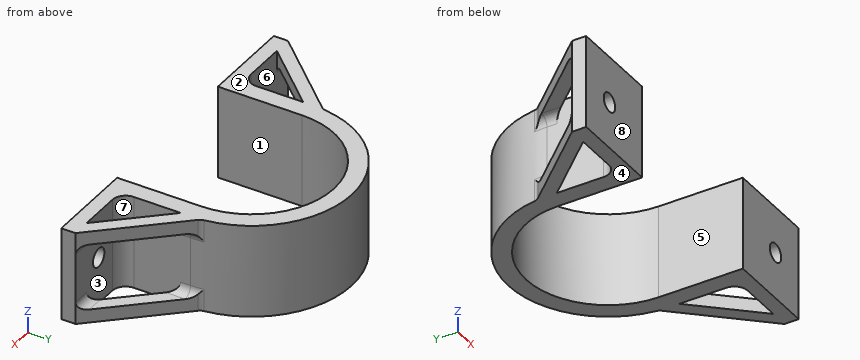
Autodesk Inventor part; units mm, degrees
ref_plane "YZ Plane" through (0, 0, 0) normal (1, 0, 0) x (0, 1, 0)
ref_plane "XZ Plane" through (0, 0, 0) normal (0, 1, 0) x (-1, 0, 0)
ref_plane "XY Plane" through (0, 0, 0) normal (0, 0, 1) x (1, 0, 0)
sketch "Эскиз1" plane through (0, 0, 0) normal (0, 0, 1) x (1, 0, 0)
  arc A0 (18.5, 0) -> (-18.5, 0) centre (0, 0) ccw
  line L0 (-22.5, 0) -> (22.5, 0)
  arc A1 (22.5, 0) -> (-22.5, 0) centre (0, 0) ccw
  line L1 (-22.5, 0) -> (-22.5, -12.8)
  line L2 (-22.5, -19) -> (-35.5, -19)
  line L3 (-35.5, -19) -> (-35.5, -15.8)
  line L4 (-35.5, -15.8) -> (-25.5, -15.8)
  arc A2 (-25.5, -15.8) -> (-22.5, -12.8) centre (-25.5, -12.8) ccw
  line L5 (-18.5, 0) -> (-18.5, -19)
  line L6 (-18.5, -19) -> (-22.5, -19)
  line L7 (0, 0) -> (0, 6.7823)
  line L8 (22.5, 0) -> (22.5, -12.8)
  line L9 (22.5, -19) -> (35.5, -19)
  line L10 (35.5, -19) -> (35.5, -15.8)
  line L11 (35.5, -15.8) -> (25.5, -15.8)
  arc A3 (22.5, -12.8) -> (25.5, -15.8) centre (25.5, -12.8) ccw
  line L12 (18.5, 0) -> (18.5, -19)
  line L13 (18.5, -19) -> (22.5, -19)
  dimension "d0" = 37
  dimension "d1" = 45
  dimension "d2" = 13
  dimension "d3" = 3.2
  dimension "d4" = 3
extrude "Выдавливание1" add sketch "Эскиз1" along normal blind 15 contours A0 L0 A1 | L0 L8 A3 L11 L10 L9 L13 L12 | L5 L6 L2 L3 L4 A2 L1 L0
sketch "Эскиз2" plane through (-35.5, -15.8, 0) normal (0, 1, 0) x (1, 0, 0)
  line L0 (71, 0) -> (61, 0)
  line L1 (61, 0) -> (61, -15)
  line L2 (71, -15) -> (61, -15)
  line L3 (71, 0) -> (71, -15)
  line L4 (71, -7.5) -> (0, -7.5)
  line L5 (0, 0) -> (0, -15)
  line L6 (10, 0) -> (0, 0)
  line L7 (10, 0) -> (10, -15)
  line L8 (10, -15) -> (0, -15)
  line L9 (5, -15) -> (5, 0)
  circle A0 centre (5, -7.5) radius 2.1
  line L10 (35.5, 0) -> (35.5, -25.4)
  circle A1 centre (66, -7.5) radius 2.1
  dimension "d7" = 4.2
extrude "Выдавливание2" cut sketch "Эскиз2" against normal blind 20 contours A1 L4 | L4 A1 | A0 L9 L4 | L4 L9 A0 | L9 A0 L4 | L4 A0 L9
sketch "Эскиз3" plane through (0, 0, 15) normal (0, 0, 1) x (1, 0, 0)
  line L0 (35.5, -15.8) -> (39.0359, -15.8)
  line L1 (22.5, 0) -> (37, -15.8)
  line L2 (21.3948, -1.0142) -> (35.8948, -16.8142)
  line L3 (22.3766, 2.3529) -> (39.0359, -15.8)
  line L4 (-18.5, -19) -> (-18.5, 0)
  arc A0 (18.5, 0) -> (-18.5, 0) centre (0, 0) ccw
  line L5 (18.5, 0) -> (18.5, -19)
  line L6 (18.5, -19) -> (35.5, -19)
  line L7 (35.5, -19) -> (35.5, -15.8)
  line L8 (35.5, -15.8) -> (25.5, -15.8)
  arc A1 (22.5, -12.8) -> (25.5, -15.8) centre (25.5, -12.8) ccw
  line L9 (22.5, -12.8) -> (22.5, 0)
  arc A2 (22.5, 0) -> (-22.5, 0) centre (0, 0) ccw
  line L10 (-22.5, 0) -> (-22.5, -12.8)
  arc A3 (-25.5, -15.8) -> (-22.5, -12.8) centre (-25.5, -12.8) ccw
  line L11 (-25.5, -15.8) -> (-35.5, -15.8)
  line L12 (-35.5, -15.8) -> (-35.5, -19)
  line L13 (-35.5, -19) -> (-18.5, -19)
  line L14 (39.0359, -15.8) -> (35.5, -15.8)
  line L15 (35.5, -15.8) -> (35.5, -19)
  line L16 (35.5, -19) -> (39.0359, -19)
  line L17 (39.0359, -19) -> (39.0359, -15.8)
  line L18 (0, 0) -> (0, 30.1625)
  line L19 (-35.5, -15.8) -> (-39.0359, -15.8)
  line L20 (-22.5, 0) -> (-37, -15.8)
  line L21 (-21.3948, -1.0142) -> (-35.8948, -16.8142)
  line L22 (-22.3766, 2.3529) -> (-39.0359, -15.8)
  line L23 (-18.5, 0) -> (-18.5, -19)
  line L24 (-18.5, -19) -> (-35.5, -19)
  line L25 (-35.5, -19) -> (-35.5, -15.8)
  line L26 (-35.5, -15.8) -> (-25.5, -15.8)
  arc A4 (-25.5, -15.8) -> (-22.5, -12.8) centre (-25.5, -12.8) ccw
  line L27 (-22.5, -12.8) -> (-22.5, 0)
  line L28 (-39.0359, -15.8) -> (-35.5, -15.8)
  line L29 (-35.5, -15.8) -> (-35.5, -19)
  line L30 (-35.5, -19) -> (-39.0359, -19)
  line L31 (-39.0359, -19) -> (-39.0359, -15.8)
  point P0 (22.5, -2.2185)
  point P1 (34.9641, -15.8)
  point P2 (35.5, -16.384)
  point P3 (-34.9641, -15.8)
  point P4 (-22.5, -2.2185)
  dimension "d11" = 1.5
  dimension "d12" = 1.5
extrude "Выдавливание3" add sketch "Эскиз3" along normal blind 3 contours L8 L2 L9 L1 L0 | L0 L17 L16 L7 | L7 L2 L8 | L1 A2 L3 L0 | L7 L6 L5 A0 L18 A2 L9 A1 L8 L2 | L18 A0 L4 L13 L12 L21 L11 A3 L10 A2 | A2 L20 L19 L22 | L10 L21 L11 L19 L20 | L19 L12 L30 L31 | L21 L12 L11
sketch "Эскиз4" plane through (0, 0, 0) normal (0, 0, -1) x (-1, 0, 0)
  line L0 (18.5, -19) -> (18.5, 0)
  line L1 (35.5, -19) -> (18.5, -19)
  line L2 (35.5, -15.8) -> (35.5, -19)
  line L3 (25.5, -15.8) -> (35.5, -15.8)
  arc A0 (22.5, -12.8) -> (25.5, -15.8) centre (25.5, -12.8) ccw
  line L4 (22.5, 0) -> (22.5, -12.8)
  arc A1 (22.5, 0) -> (-22.5, 0) centre (0, 0) ccw
  line L5 (-22.5, -12.8) -> (-22.5, 0)
  arc A2 (-25.5, -15.8) -> (-22.5, -12.8) centre (-25.5, -12.8) ccw
  line L6 (-35.5, -15.8) -> (-25.5, -15.8)
  line L7 (-35.5, -19) -> (-35.5, -15.8)
  line L8 (-18.5, -19) -> (-35.5, -19)
  line L9 (-18.5, 0) -> (-18.5, -19)
  arc A3 (18.5, 0) -> (-18.5, 0) centre (0, 0) ccw
  line L10 (-35.5, -19) -> (-35.5, -15.8)
  line L11 (-35.5, -15.8) -> (-34.9641, -15.8)
  line L12 (-22.5, -2.2185) -> (-34.9641, -15.8)
  line L13 (-22.5, -2.2185) -> (-22.5, 0)
  arc A4 (-22.3766, 2.3529) -> (-22.5, 0) centre (0, 0) ccw
  line L14 (-39.0359, -15.8) -> (-22.3766, 2.3529)
  line L15 (-39.0359, -19) -> (-39.0359, -15.8)
  line L16 (-35.5, -19) -> (-39.0359, -19)
  line L17 (35.5, -15.8) -> (35.5, -19)
  line L18 (39.0359, -19) -> (35.5, -19)
  line L19 (39.0359, -15.8) -> (39.0359, -19)
  line L20 (22.3766, 2.3529) -> (39.0359, -15.8)
  arc A5 (22.5, 0) -> (22.3766, 2.3529) centre (0, 0) ccw
  line L21 (22.5, 0) -> (22.5, -2.2185)
  line L22 (34.9641, -15.8) -> (22.5, -2.2185)
  line L23 (34.9641, -15.8) -> (35.5, -15.8)
  point P0 (-22.3766, 2.3529)
extrude "Выдавливание4" add sketch "Эскиз4" along normal blind 3 contours L0 A3 L9 L8 L7 L6 A2 L5 A1 L4 A0 L3 L2 L1 | L2 L3 L22 L4 A1 L20 L19 L18 | L16 L15 L14 A1 L5 L12 L6 L7
sketch "Эскиз5" plane through (0, 0, 15) normal (0, 0, -1) x (-1, 0, 0)
  line L0 (-35.5, -19) -> (-35.5, -15.8)
  line L1 (-35.5, -15.8) -> (-34.9641, -15.8)
  line L2 (-22.5, -2.2185) -> (-34.9641, -15.8)
  line L3 (-22.5, -2.2185) -> (-22.5, 0)
  arc A0 (-22.3766, 2.3529) -> (-22.5, 0) centre (0, 0) ccw
  line L4 (-39.0359, -15.8) -> (-22.3766, 2.3529)
  line L5 (-39.0359, -19) -> (-39.0359, -15.8)
  line L6 (-35.5, -19) -> (-39.0359, -19)
  line L7 (35.5, -15.8) -> (35.5, -19)
  line L8 (39.0359, -19) -> (35.5, -19)
  line L9 (39.0359, -15.8) -> (39.0359, -19)
  line L10 (22.3766, 2.3529) -> (39.0359, -15.8)
  arc A1 (22.5, 0) -> (22.3766, 2.3529) centre (0, 0) ccw
  line L11 (22.5, 0) -> (22.5, -2.2185)
  line L12 (34.9641, -15.8) -> (22.5, -2.2185)
  line L13 (34.9641, -15.8) -> (35.5, -15.8)
  line L14 (39.0359, -15.8) -> (-39.0359, -15.8)
  line L15 (-18.5, -19) -> (-39.0359, -19)
extrude "Выдавливание5" add sketch "Эскиз5" along normal up to surface (15 mm away) contours L6 L5 L14 L0 | L14 L9 L8 L7
fillet "Сопряжение1" radius 2 16 edges at (-37, -15.8, 15) (-37, -15.8, 0) (-22.5, -1.1092, 0) (-22.4691, 1.1781, 0) (-22.5, -1.1092, 15) (-22.4691, 1.1781, 15) (22.3766, 2.3529, 16.5) (22.3766, 2.3529, -1.5) (22.5, -1.1092, 0) (22.4691, 1.1781, 0) (37, -15.8, 0) (37, -15.8, 15) (22.4691, 1.1781, 15) (22.5, -1.1092, 15) (-22.3766, 2.3529, 16.5) (-22.3766, 2.3529, -1.5)
properties part number "доп крепл мотора 25-26"
Here's how the part is built. I have some questions about the finished solid (model axes, mm). Face numbers are marked on the shaded views. A direction names the side the tool comes from. Give positions to 0.01 mm unless a question says otherwise; leave off trailing zeros. Loops run counter-clockwise (first coordinate to the right, second up) from the corner with the lowest first, then second, coordinate; pieces in that order, holes last. Notation, with made-up numbers: M -39.5,63 L 2.5,63 A19 ccw 2.5,77 Z; hole C -27.5,66 d2. An arc over 180 degrees is marked long. Put each result on its own line as item: value. Start each with the question number.
(1) I want a section at C-C on z = 16.5. Please give me the cut outline in (x, y).
(2) I need wall thicknesses on line 1 along X through (y, z) = (-17.15, 7.5); line 2 along Z through (x, y) = (-30.5, -17.95); line 3 along X through (y, z) = (-11.5, 2). Which ranges of each line are inside material? Lowest first, please. Write a range as [from, to].
(3) I want a section at A-A on z = 7.5. Please give me the cut outline in (x, y), then the cut area to 3 significant figures.
(4) I want a section at B-B on y = -9.5. Please give me the cut outline in (x, z), then the cut area to 3 significant figures.
(5) Will these pins go through, and if not, where does the flat tip stop? pin 1 Ø5 at (y, z) = (-6, 15) entering from +X; pin 2 Ø6 at (y, z) = (-5, 14.5) entering from -X; pin 3 Ø2 at (y, z) = (-7.5, 12) entering from -X.
(6) I want a section at D-D on x = -30.5. Please give me the cut outline in (y, z), then the cut area to 3 significant figures.
(7) If we mould it in two halves opening along Z, with no side actions, what happens to the marked faces 1, 2, 3 and 4? For each: +Z half, -Z half, draft (parallel to the pull), parting line (faces both ways), or undercut.
(8) For the marked faces 5, 6, 7 and 8, which set-ups out of +Z, -Z, +X, -X, +Y, -Y let a thin tool reach every point of the face, with its end or its side?
Answer block:
1. outline: M -39.04,-19 L -18.5,-19 L -18.5,0 A18.5 cw 18.5,0 L 18.5,-19 L 39.04,-19 L 39.04,-15.8 L 22.81,1.88 A2 cw 22.3,2.97 A22.5 ccw -22.3,2.97 A2 cw -22.81,1.88 L -39.04,-15.8 Z; hole M -34.96,-15.8 L -25.5,-15.8 A3 ccw -22.5,-12.8 L -22.5,-2.22 Z; hole M 22.5,-12.8 A3 ccw 25.5,-15.8 L 34.96,-15.8 L 22.5,-2.22 Z
2. line 1: [-39.04, -32.6], [-28.4, -18.5], [18.5, 28.4], [32.6, 39.04]
2. line 2: [-3, 5.4], [9.6, 18]
2. line 3: [-22.5, -18.5], [18.5, 22.5]
3. outline: M -39.04,-19 L -32.6,-19 L -32.6,-15.8 L -39.04,-15.8 Z; M -28.4,-19 L -18.5,-19 L -18.5,0 A18.5 cw 18.5,0 L 18.5,-19 L 28.4,-19 L 28.4,-15.8 L 25.5,-15.8 A3 cw 22.5,-12.8 L 22.5,0 A22.5 ccw -22.5,0 L -22.5,-12.8 A3 cw -25.5,-15.8 L -28.4,-15.8 Z; M 32.6,-19 L 39.04,-19 L 39.04,-15.8 L 32.6,-15.8 Z
3. area: 492 mm^2
4. outline: M -33.25,-3 L -29.18,-3 L -29.18,0 L -33.25,0 Z; M -33.25,15 L -29.18,15 L -29.18,18 L -33.25,18 Z; M -22.5,-3 L -18.5,-3 L -18.5,18 L -22.5,18 Z; M 18.5,-3 L 22.5,-3 L 22.5,18 L 18.5,18 Z; M 29.18,-3 L 33.25,-3 L 33.25,0 L 29.18,0 Z; M 29.18,15 L 33.25,15 L 33.25,18 L 29.18,18 Z
4. area: 217 mm^2
5. pin 1: x = 32.34
5. pin 2: x = -31.84
5. pin 3: x = -22.5
6. outline: M -19,-3 L -15.8,-3 L -15.8,5.4 L -19,5.4 Z; M -19,9.6 L -15.8,9.6 L -15.8,18 L -19,18 Z; M -10.94,-3 L -6.5,-3 L -6.5,0 L -10.94,0 Z; M -10.94,15 L -6.5,15 L -6.5,18 L -10.94,18 Z
6. area: 80.4 mm^2
7. face 1: draft
7. face 2: +Z half
7. face 3: undercut
7. face 4: -Z half
8. face 5: +Z, -Z, -Y
8. face 6: none
8. face 7: +Z, -Z
8. face 8: +Z, -Z, +X, -X, -Y
